from build123d import *

# Parameters (mm, degrees)
SKETCH1_W           = 92
SKETCH1_H           = 122
BOSS_EXTRUDE1_DEPTH = 5
SKETCH2_W           = 5
SKETCH2_H           = 60
SKETCH2_W_2         = 30
SKETCH2_H_2         = 5
CUT_EXTRUDE1_DEPTH  = 6
SKETCH3_R           = 4.03
CUT_EXTRUDE2_DEPTH  = 5
SKETCH4_W           = 70
SKETCH4_H           = 9
CUT_EXTRUDE3_DEPTH  = 10


with BuildPart() as part:
    # Sketch1 → Boss-Extrude1 (new body)
    with BuildSketch(Plane(origin=(0, 0, 0), x_dir=(1, 0, 0), z_dir=(0, 1, 0))):
        Rectangle(SKETCH1_W, SKETCH1_H)
    extrude(amount=BOSS_EXTRUDE1_DEPTH)

    # Sketch2 → Cut-Extrude1 (cut, through all)
    with BuildSketch(Plane(origin=(0, 5, 0), x_dir=(1, 0, 0), z_dir=(0, 1, 0))):
        with Locations((-37.5, 0)):
            Rectangle(SKETCH2_W, SKETCH2_H)
        with Locations((37.5, 0)):
            Rectangle(SKETCH2_W, SKETCH2_H)
        with Locations((0, 52.5)):
            Rectangle(SKETCH2_W_2, SKETCH2_H_2)
        with Locations((0, -52.5)):
            Rectangle(SKETCH2_W_2, SKETCH2_H_2)
    extrude(amount=-CUT_EXTRUDE1_DEPTH, mode=Mode.SUBTRACT)

    # Sketch3 → Cut-Extrude2 (cut)
    with BuildSketch(Plane(origin=(0, 5, 0), x_dir=(1, 0, 0), z_dir=(0, 1, 0))):
        with Locations(Location((0, 0, 0), (0, 0, 270))):  # turned: the seam where the file's is
            Circle(SKETCH3_R)
        with Locations(Location((-20, 0, 0), (0, 0, 270))):  # turned: the seam where the file's is
            Circle(SKETCH3_R)
        with Locations(Location((20, 0, 0), (0, 0, 270))):  # turned: the seam where the file's is
            Circle(SKETCH3_R)
    extrude(amount=-CUT_EXTRUDE2_DEPTH, mode=Mode.SUBTRACT)

    # Sketch4 → Cut-Extrude3 (cut)
    with BuildSketch(Plane(origin=(0, 5, 0), x_dir=(1, 0, 0), z_dir=(0, 1, 0))):
        Rectangle(SKETCH4_W, SKETCH4_H)
    extrude(amount=-CUT_EXTRUDE3_DEPTH, mode=Mode.SUBTRACT)


solid = part.part
For this review, take the finished solid that the model builds, in its own axes (mm). A direction names the side the tool comes from. Give positions to 0.01 mm unless a question says otherwise; leave off trailing zeros. Loops run counter-clockwise (first coordinate to the right, second up) from the corner with the lowest first, then second, coordinate; pieces in that order, holes last. Notation, with made-up numbers: M 51,-39 L 93,-39 A26 cw 93,-25 Z; hole C -23.75,77.5 d3. An arc over 180 degrees is marked long. Put each result on its own line as item: value. Start each with the question number.
(1) Add section A-A, the plane z = -23.5. Write out the cut boundary in (x, y), then the cut area to 3 significant figures.
(2) The part is to be moulded in two halves that separate along Z. For faces 3 (the flat face through (-46, 2, 1)), 4 (the flat face through (37, 3, -30)), 5 (the flat face through (-1, 2, 61)), say which applies: +Z half, -Z half, draft (parallel to the pull), parting line (faces both ways), or undercut.
(3) Add section B-B, the plane y = 4.1. Write out the cut boundary in (x, z).
(4) For pin 1 (1 mm diameter, centred on x = 29, z = 33, fed in from -Y), flat-tipped, find the tip position at first contact; note if it passes through.
(5) Add section C-C, the plane x = 4.5. Write out the cut boundary in (y, z).
(6) Machinability: for faces 1 (the flat face through (-40, 3, 0)), 2 (the flat face through (-1, 0, -14)), which of the approach directions +Z, -Z, +X, -X, +Y, -Y give a long, thin tool a straight path to every point of the face, cutting with its end or side? Answer none if there is none.
(7) Add section D-D, the plane z = -2. Write out the cut boundary in (x, y).
(8) Wall thickness on L1, parallel to X at y = 0.35, z = 14; L2, parallel to Z at x = 10.5, y = 0.25; L3, parallel to Z at x = 21, y = 0.45: over which ranges is each line inside the solid? List them lowest first.
Result:
1. outline: M -46,0 L -40,0 L -40,5 L -46,5 Z; M -35,0 L 35,0 L 35,5 L -35,5 Z; M 40,0 L 46,0 L 46,5 L 40,5 Z
1. area: 410 mm^2
2. face 3: draft
2. face 4: undercut
2. face 5: +Z half
3. outline: M -46,-61 L 46,-61 L 46,61 L -46,61 Z; hole M -40,-30 L -35,-30 L -35,-4.5 L 35,-4.5 L 35,-30 L 40,-30 L 40,30 L 35,30 L 35,4.5 L -35,4.5 L -35,30 L -40,30 Z; hole M -15,-55 L 15,-55 L 15,-50 L -15,-50 Z; hole M -15,50 L 15,50 L 15,55 L -15,55 Z
4. pin 1: stops at y = 0
5. outline: M 0,-61 L 5,-61 L 5,-55 L 0,-55 Z; M 0,-50 L 5,-50 L 5,-4.5 L 0,-4.5 Z; M 0,4.5 L 5,4.5 L 5,50 L 0,50 Z; M 0,55 L 5,55 L 5,61 L 0,61 Z
6. face 1: +Y, -Y
6. face 2: +Z, -Z, +X, -X, -Y
7. outline: M -46,0 L -40,0 L -40,5 L -46,5 Z; M 40,0 L 46,0 L 46,5 L 40,5 Z
8. L1: x = -46 to -40, -35 to 35, 40 to 46
8. L2: z = -61 to -55, -50 to -4.5, 4.5 to 50, 55 to 61
8. L3: z = -61 to -4.5, 4.5 to 61
